Source: CAD feature listing. Evaluate the final solid. Frame: model axes, mm. A direction names the side the tool comes from. Round coordinates to 2 decimals unless told otherwise and drop trailing zeros. Loops run counter-clockwise (first coordinate to the right, second up) from the corner with the lowest first, then second, coordinate; pieces in that order, holes last. Notation, with made-up numbers: M 17.5,48.25 L 69.5,48.25 A28 ccw 69.5,82.25 Z; hole C 15.25,76.5 d11. An arc over 180 degrees is marked long. Answer as CSV lines item,"result". Start each with the question number.
```python
from build123d import *

# Parameters (mm, degrees)
F0_W     = 43
F0_H     = 150
F1_DEPTH = 150
F2_W     = 23
F2_H     = 140
F3_DEPTH = 140
F5_DEPTH = 43.001
F7_D     = 6.7564
F9_DEPTH = 43.001


with BuildPart() as f1:
    # F0 (on Top) → F1 (new body)
    with BuildSketch(Plane.XY):
        Rectangle(F0_W, F0_H)
    extrude(amount=F1_DEPTH)

    # F2 (on face) → F3 (cut)
    with BuildSketch(Plane.XY.offset(150)):
        with Locations((0, 5)):
            Rectangle(F2_W, F2_H)
    extrude(amount=-F3_DEPTH, mode=Mode.SUBTRACT)

    # F4 (on face) → F5 (cut, through all)
    with BuildSketch(Plane.YZ.offset(21.5)):
        with BuildLine():
            Line((75, 150), (-75, 150))
            ThreePointArc((-75, 150), (31.066017178, 106.066017178), (75, 0))
            Line((75, 0), (75, 150))
        make_face()
    extrude(amount=-F5_DEPTH, mode=Mode.SUBTRACT)

    # F7 (through all)
    with Locations(Plane.YZ.offset(21.5)):
        with Locations((-55, 20)):
            Hole(F7_D / 2)

    # F8 (on face) → F9 (cut, through all)
    with BuildSketch(Plane.YZ.offset(21.5)):
        with BuildLine():
            Line((-5, 113.9230484541), (-15, 96.6025403784))
            ThreePointArc((-15, 96.6025403784), (21.6025403784, 60), (35, 10))
            Line((35, 10), (55, 10))
            Line((55, 10), (54.5824738826, 20.0015968781))
            Line((54.5824738826, 20.0015968781), (39.3695273594, 44.7419308441))
            Line((39.3695273594, 44.7419308441), (48.8576662103, 47.9002881935))
            Line((48.8576662103, 47.9002881935), (45.3067125626, 57.248589012))
            Line((45.3067125626, 57.248589012), (23.0601812824, 75.9196819812))
            Line((23.0601812824, 75.9196819812), (31.0656523081, 81.9123803431))
            Line((31.0656523081, 81.9123803431), (24.7445969083, 89.6612033914))
            Line((24.7445969083, 89.6612033914), (-2.2593001309, 100.3526678075))
            Line((-2.2593001309, 100.3526678075), (3.4443998572, 108.5665466991))
            ThreePointArc((3.4443998572, 108.5665466991), (-0.7219789397, 111.3327982865), (-5, 113.9230484541))
        make_face()
    extrude(amount=-F9_DEPTH, mode=Mode.SUBTRACT)


solid = f1.part
```
1) Section A-A, the plane y = -11. Return loops of the section in (x, z).
2) Access query for faces 1 (the flat face through (0, -65, 81)), 2 (the flat face through (16.57, 34.339, 66.453)), 3 (the flat face through (0, -75, 74)). Directions: +Z, -Z, +X, -X, +Y, -Y. A direction counts if a zero-diameter tool reaches every point of the face in a straight line with its end or side. Return the directions, or none.
3) Contact query for flat-ended pins moving along their axis: pin 1 Ø6 at (x, y) = (-0.5, -35) entering from +Z; pin 2 Ø4 at (x, z) = (-4, 71.5) entering from +Y; pin 3 Ø13 at (x, y) = (-7.5, -9) entering from +Z. Output: stop coordinate, or through.
4) Section B-B, the plane z = 87. Return loops of the section in (x, y).
5) Ray query, line 1 along X through (y, z) = (-60, 130); line 2 along Z through (x, y) = (-7, -40); line 3 along Y through (x, z) = (-10, 42.5). Return the intervals inside material, ascending.
6) Section D-D, the plane y = -40. Return loops of the section in (x, z), and give its area (3 significant figures).
7) Mould query, pull axis Z, two halves, no side actions, for faces 4 (the flat face through (-16.43, 54.794, 14.931)), 5 (the cylindrical face through (14.63, 29.89, 107.23)), 6 (the flat face through (-16.43, -9.93, 105.384)), 7 (the flat face through (21.5, -18, 57)). Classes: pulls with the +Z half, pulls with the -Z half, needs draft (parallel to the pull), parting line crosses it, or undercut.
8) Section C-C, the plane x = -8.5. Return loops of the section in (y, z), and give its area (3 significant figures).
Findings below:
1,outline,"M -21.5,0 L 21.5,0 L 21.5,94.17 L 11.5,94.17 L 11.5,10 L -11.5,10 L -11.5,94.17 L -21.5,94.17 Z; M -21.5,103.53 L -11.5,103.53 L -11.5,135.66 L -21.5,135.66 Z; M 11.5,103.53 L 21.5,103.53 L 21.5,135.66 L 11.5,135.66 Z"
2,face 1,"+Z, +Y"
2,face 2,"+X, -X"
2,face 3,"+Z, -Z, +X, -X, -Y"
3,pin 1,"z = 10"
3,pin 2,"y = -65"
3,pin 3,"z = 137.09"
4,outline,"M -21.5,-75 L 21.5,-75 L 21.5,-1.2 L 11.5,-1.2 L 11.5,-65 L -11.5,-65 L -11.5,-1.2 L -21.5,-1.2 Z; M -21.5,26.92 L -11.5,26.92 L -11.5,47.19 L -21.5,47.19 Z; M 11.5,26.92 L 21.5,26.92 L 21.5,47.19 L 11.5,47.19 Z"
5,line 1,"-21.5 to -11.5, 11.5 to 21.5"
5,line 2,"0 to 10"
5,line 3,"-75 to -65"
6,outline,"M -21.5,0 L 21.5,0 L 21.5,145.86 L 11.5,145.86 L 11.5,10 L -11.5,10 L -11.5,145.86 L -21.5,145.86 Z"
6,area,"3,150 mm²"
7,face 4,"undercut"
7,face 5,"pulls with the +Z half"
7,face 6,"undercut"
7,face 7,"needs draft"
8,outline,"M -75,0 L 75,0 A150 ccw 74.67,10 L -65,10 L -65,149.67 A150 ccw -75,150 Z"
8,area,"2,900 mm²"
